Here's the drawing with two shaded views (mm, measured from the low corner). I have some questions. A direction names the side the tool comes from. Coordinates: 2 decimals unless noted, no trailing zeros. Write each loop counter-clockwise with the first axis right and the second up, starting at its lowest first coordinate (ties: lowest second). Pieces come first, ordered by that corner, then holes. Notation, with made-up numbers: M 85.5,39 L 105.5,39 A30 ccw 105.5,78 Z; hole C 24.5,6.5 d5. An arc over 180 degrees is marked long. Answer as CSV lines item,"result". Start each with the question number.
Item 1: If I drill on line 1 along Y through (x, z) = (8.5, 10); line 2 along Y through (x, z) = (14, 10); line 3 along Y through (x, z) = (28.5, 14), over which ranges is the centre line in solid material (lowest first)? Write a range as [from, to].
Item 2: I'm going to push a flat-ended pin straight in: P1, Ø18, axis at x = 30, y = 140, coming from the -Z side. Where does the tip first touch, or does it pass through?
Item 3: On a 3-axis mill with a long thin cutter (end or side, diameter ignored), from which of +Z, -Z, +X, -X, +Y, -Y can I reach the whole of each face in a straight line? I mean the marked faces 5 and 6. Say none if no direction works.
Item 4: Suppose I cut it at B-B, the plane z = 16.5. Write out the boundary of the cut face in (x, y).
Item 5: We'd pull the mould along Y, two halves only. Please class the marked faces 1, 2, 3 and 4: +Y half, -Y half, draft (parallel to the pull), parting line (faces both ways), or undercut.
Item 6: Suppose I cut it at A-A, the plane x = 30. Write out the boundary of the cut face in (y, z).
Item 7: Suppose I cut it at C-C, the plane y = 220. Write out the boundary of the cut face in (x, z), and give its area (3 significant figures).
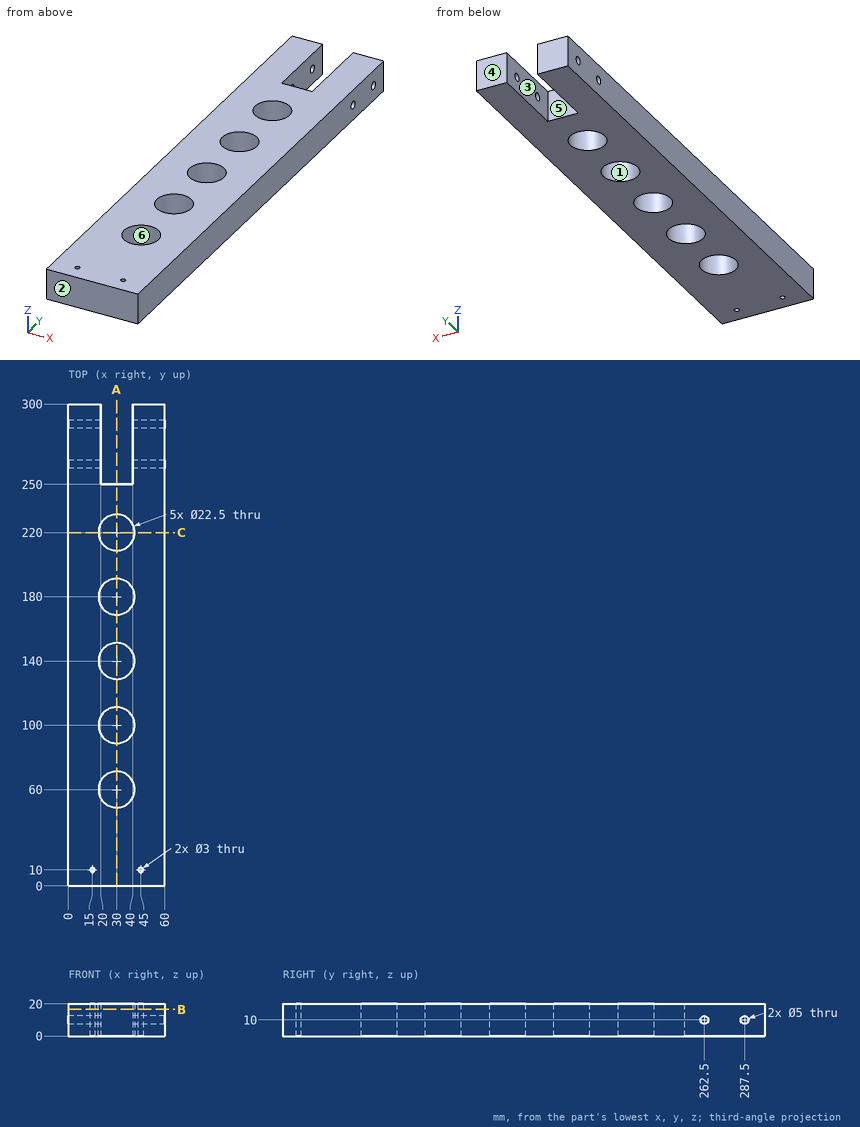
Ans:
1,line 1,"y = [0, 260], [265, 285], [290, 300]"
1,line 2,"y = [0, 8.88], [11.12, 260], [265, 285], [290, 300]"
1,line 3,"y = [0, 48.85], [71.15, 88.85], [111.15, 128.85], [151.15, 168.85], [191.15, 208.85], [231.15, 250]"
2,P1,"passes through"
3,face 5,"+Z, -Z, +Y"
3,face 6,"+Z, -Z"
4,outline,"M 0,0 L 60,0 L 60,300 L 40,300 L 40,250 L 20,250 L 20,300 L 0,300 Z; hole C 15,10 d3; hole C 30,60 d22.5; hole C 30,100 d22.5; hole C 30,140 d22.5; hole C 30,180 d22.5; hole C 30,220 d22.5; hole C 45,10 d3"
5,face 1,"undercut"
5,face 2,"-Y half"
5,face 3,"draft"
5,face 4,"+Y half"
6,outline,"M 0,0 L 48.75,0 L 48.75,20 L 0,20 Z; M 71.25,0 L 88.75,0 L 88.75,20 L 71.25,20 Z; M 111.25,0 L 128.75,0 L 128.75,20 L 111.25,20 Z; M 151.25,0 L 168.75,0 L 168.75,20 L 151.25,20 Z; M 191.25,0 L 208.75,0 L 208.75,20 L 191.25,20 Z; M 231.25,0 L 250,0 L 250,20 L 231.25,20 Z"
7,outline,"M 0,0 L 18.75,0 L 18.75,20 L 0,20 Z; M 41.25,0 L 60,0 L 60,20 L 41.25,20 Z"
7,area,"750 mm^2"
